```python
from build123d import *

# Parameters (mm, degrees)
F0_R     = 9.525
F1_DEPTH = 25.4
F3_DEPTH = 25.401
F4_DEPTH = 11.0998
F6_DEPTH = 9.525
F7_R     = 0.61321


with BuildPart() as f1:
    # F0 (on Front) → F1 (new body)
    with BuildSketch(Plane.XZ):
        Circle(F0_R)
    extrude(amount=F1_DEPTH)

    # F2 (on Front) → F3 (cut, through all)
    with BuildSketch(Plane.XZ):
        with BuildLine():
            ThreePointArc((4.7625, 0), (3.367596, 3.367596), (0, 4.7625))
            ThreePointArc((0, 4.7625), (-3.367596, 3.367596), (-4.7625, 0))
            ThreePointArc((-4.7625, 0), (-3.367596, -3.367596), (0, -4.7625))
            ThreePointArc((0, -4.7625), (3.367596, -3.367596), (4.7625, 0))
        make_face()
    extrude(amount=F3_DEPTH, mode=Mode.SUBTRACT)

    # F2 (on Front) → F4 (cut)
    with BuildSketch(Plane.XZ):
        with BuildLine():
            ThreePointArc((0, -4.7625), (-3.367596, -3.367596), (-4.7625, 0))
            Line((-4.7625, 0), (-4.7625, -4.7625))
            Line((-4.7625, -4.7625), (0, -4.7625))
        make_face()
        with BuildLine():
            ThreePointArc((-4.7625, 0), (-3.367596, 3.367596), (0, 4.7625))
            Line((0, 4.7625), (-4.7625, 4.7625))
            Line((-4.7625, 4.7625), (-4.7625, 0))
        make_face()
        with BuildLine():
            Line((4.7625, 0), (4.7625, 4.7625))
            Line((4.7625, 4.7625), (0, 4.7625))
            ThreePointArc((0, 4.7625), (3.367596, 3.367596), (4.7625, 0))
        make_face()
        with BuildLine():
            Line((4.7625, -4.7625), (4.7625, 0))
            ThreePointArc((4.7625, 0), (3.367596, -3.367596), (0, -4.7625))
            Line((0, -4.7625), (4.7625, -4.7625))
        make_face()
    extrude(amount=F4_DEPTH, mode=Mode.SUBTRACT)

    # F5 (on face) → F6 (cut)
    with BuildSketch(Plane.XZ.offset(25.4)):
        Polygon((3.65125, -6.324151), (7.3025, 0), (3.65125, 6.324151), (-3.65125, 6.324151), (-7.3025, 0), (-3.65125, -6.324151), align=None)
    extrude(amount=-F6_DEPTH, mode=Mode.SUBTRACT)

    # F7
    f7_edges = [f1.edges().sort_by_distance(p)[0] for p in [
        (-9.525, 0, 0),
    ]]
    fillet(f7_edges, radius=F7_R)


solid = f1.part
```
The model under review builds one solid part; all positions refer to its coordinate system, in mm. A direction names the side the tool comes from. Round coordinates to 2 decimals unless told otherwise and drop trailing zeros. Answer in a Markdown table with one row per item.
(1) Clearance check with flat-ended pins moving along their axes: P1, Ø6.5, axis at x = 1.5, z = 1, coming from the -Y side (3 decimals); P2, Ø3, axis at y = -6, z = -2, coming from the -X side; P3, Ø1, axis at x = 6.5, y = -11, coming from the +Z side. State where each tip first meets the part, or that it passes through.
Result set:
| item | result |
|---|---|
| P1 | stops at y = -15.875 |
| P2 | stops at x = -9.51 |
| P3 | stops at z = 7.4 |
(2) For line 1 (X direction, y = -20.5, z = 4.5); line 2 (X direction, y = -17.25, z = 4); line 3 (Z direction, x = -8.25, y = -5), list the stretches that pass through material, from the lowest coordinate up. Write a range as from..to.
Result set:
| item | result |
|---|---|
| line 1 | x = -8.39..-4.7, 4.7..8.39 |
| line 2 | x = -8.64..-4.99, 4.99..8.64 |
| line 3 | z = -4.76..4.76 |
(3) Machinability: for faces 4 (the face through (4.762, -5, 0)), 5 (the face through (0, 0, -6)), 6 (the face through (5.45, -20.7, -3.21)), which of the approach directions +Z, -Z, +X, -X, +Y, -Y give a long, thin tool a straight path to every point of the face, cutting with its end or side? Answer none if there is none.
Result set:
| item | result |
|---|---|
| face 4 | +Y |
| face 5 | +Z, -Z, +X, -X, +Y |
| face 6 | -Y |
(4) Mouldability with a two-part tool opening along Z and no side actions: class faces 1 (the face through (6.2, -25.4, 2.3)), 2 (the face through (0, -5, -4.762)), 3 (the face through (-7.559, -12.833, -5.796)) as released by +Z, released by -Z, zero draft, split by the parting line, or undercut.
Result set:
| item | result |
|---|---|
| face 1 | zero draft |
| face 2 | undercut |
| face 3 | split by the parting line |
